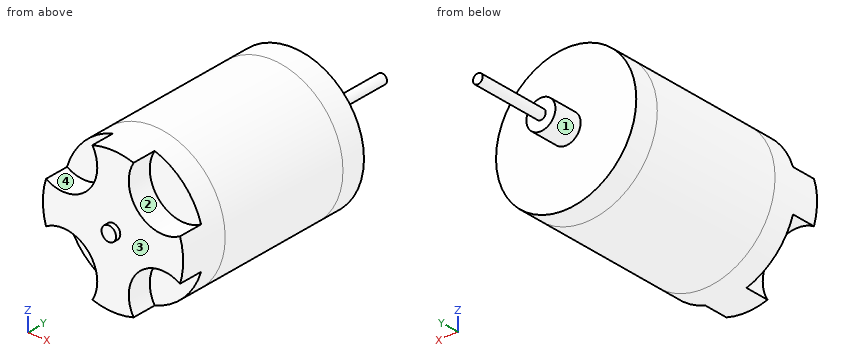
Autodesk Fusion 360 part; units mm, degrees
sketch "Sketch1" plane through (0, 0, 0) normal (0, 1, 0) x (1, 0, 0)
  circle A0 centre (0, 0) radius 14.5
  dimension "d1" = 29
extrude "Extrude1" add sketch "Sketch1" along normal blind 5
sketch "Sketch2" plane through (0, 0, 0) normal (0, -1, 0) x (1, 0, 0)
  circle A0 centre (0, 0) radius 14.5
  circle A1 centre (0, 0) radius 1.5
  circle A2 centre (0, 0) radius 14.5
  dimension "d4" = 3
extrude "Extrude2" add sketch "Sketch2" along normal blind 5 contours A0 A2 | A1
sketch "Sketch3" plane through (0, -5, 0) normal (0, -1, 0) x (1, 0, 0)
  circle A0 centre (0, 0) radius 14.5
  line L0 (0, 0) -> (10.253, 10.253)
  line L1 (0, 0) -> (14.5, 0) construction
  line L2 (0, 0) -> (10.253, -10.253)
  line L3 (0, 0) -> (-10.253, -10.253)
  line L4 (0, 0) -> (-10.253, 10.253)
  circle A1 centre (-10.253, -10.253) radius 7
  circle A2 centre (10.253, -10.253) radius 7
  circle A3 centre (10.253, 10.253) radius 7
  circle A4 centre (-10.253, 10.253) radius 7
  dimension "d7" = 45
  dimension "d8" = 14
  dimension "d9" = 14
  dimension "d10" = 14
  dimension "d11" = 14
extrude "Extrude3" cut sketch "Sketch3" against normal blind 5 contours A0 L0 A3 | A0 L2 A2 | A0 L0 A3 | A0 L2 A2 | A0 L4 A4 | A0 L3 A1 | A0 L3 A1 | A0 L4 A4
sketch "Sketch4" plane through (0, -5, 0) normal (0, -1, 0) x (1, 0, 0)
  arc A0 (-4.2549, -13.8617) -> (-13.8617, -4.2549) centre (-10.253, -10.253) ccw
  arc A1 (-4.2549, -13.8617) -> (4.2549, -13.8617) centre (0, 0) ccw
  arc A2 (13.8617, -4.2549) -> (4.2549, -13.8617) centre (10.253, -10.253) ccw
  arc A3 (13.8617, -4.2549) -> (13.8617, 4.2549) centre (0, 0) ccw
  arc A4 (4.2549, 13.8617) -> (13.8617, 4.2549) centre (10.253, 10.253) ccw
  arc A5 (4.2549, 13.8617) -> (-4.2549, 13.8617) centre (0, 0) ccw
  arc A6 (-13.8617, 4.2549) -> (-4.2549, 13.8617) centre (-10.253, 10.253) ccw
  arc A7 (-13.8617, 4.2549) -> (-13.8617, -4.2549) centre (0, 0) ccw
  circle A8 centre (0, 0) radius 1.5
  dimension "d14" = 3
extrude "Extrude4" add sketch "Sketch4" along normal blind 1 contours A8
sketch "Sketch5" plane through (0, 5, 0) normal (0, 1, 0) x (-1, 0, 0)
  circle A0 centre (0, 0) radius 14.5
  circle A1 centre (0, 0) radius 14.5
extrude "Extrude5" add sketch "Sketch5" along normal blind 28
sketch "Sketch6" plane through (0, 33, 0) normal (0, 1, 0) x (-1, 0, 0)
  circle A0 centre (0, 0) radius 14.5
  circle A1 centre (0, 0) radius 14.5
extrude "Extrude6" add sketch "Sketch6" along normal blind 5
sketch "Sketch7" plane through (0, 38, 0) normal (0, 1, 0) x (-1, 0, 0)
  circle A0 centre (0, 0) radius 14.5
  line L0 (0, 0) -> (10.253, -10.253)
  line L1 (0, 0) -> (14.5, 0) construction
  line L2 (0, 0) -> (-10.253, -10.253)
  line L3 (0, 0) -> (14.5, 0) construction
  line L4 (0, 0) -> (-10.253, 10.253)
  line L5 (-10.253, 10.253) -> (-6.7175, 6.7175)
  line L6 (-10.253, -10.253) -> (-6.7175, -6.7175)
  line L7 (10.253, -10.253) -> (6.7175, -6.7175)
  line L8 (10.253, 10.253) -> (8.8388, 8.8388)
  circle A1 centre (0, 0) radius 3.5
  circle A2 centre (0, 0) radius 12.5
  circle A3 centre (0, 0) radius 3
  dimension "d21" = 45
  dimension "d22" = 14.5
  dimension "d23" = 135
  dimension "d25" = 5
  dimension "d26" = 5
  dimension "d27" = 5
  dimension "d28" = 2
  dimension "d29" = 7
  dimension "d30" = 6
extrude "Extrude7" add sketch "Sketch7" along normal blind 6 contours L0 L2 A3 | L0 L4 A3 | L2 L4 A3
sketch "Sketch8" plane through (0, 44, 0) normal (0, 1, 0) x (-1, 0, 0)
  circle A0 centre (0, 0) radius 3
  circle A1 centre (0, 0) radius 1
  dimension "d33" = 2
extrude "Extrude8" add sketch "Sketch8" along normal blind 15 contours A1
equation "d8 = 0.7 cm * 2"
equation "d23 = 90 deg + 45 deg"
Read the model definition and answer for the solid it produces. Units are mm, in the model's axes. Face numbers are marked on the shaded views. Round coordinates to 2 decimals unless told otherwise and drop trailing zeros. Loops run counter-clockwise (first coordinate to the right, second up) from the corner with the lowest first, then second, coordinate; pieces in that order, holes last. Notation, with made-up numbers: (-5.5, 26) -> (1.5, 26) arc R20 cw to (1.5, 55) -> close; hole circle Ø10 at (24, 57). An arc over 180 degrees is marked (long way). One line per item, written item: value.
1) Flat-ended cylindrical pins translate along their axes: P1, Ø5.5, axis at x = -9, z = 9, coming from the -Y side; P2, Ø8.5, axis at x = 6.5, z = 7, coming from the -Y side; P3, Ø4, axis at x = -9, y = 8, coming from the -Z side. Find the tip coordinate at first contact, or state that the pin passes through.
Answer list:
P1: stops at y = 0
P2: stops at y = -5
P3: stops at z = -12.7
2) The mould has two halves that part along X. Classify the marked faces 1, 2, 3 and 4: pulls with the +X half, pulls with the -X half, needs draft (parallel to the pull), parting line crosses it, or undercut.
Answer list:
face 1: parting line crosses it
face 2: undercut
face 3: needs draft
face 4: undercut
3) A cutting plane is placed at C-C (y = 37). Determine the outline of the cut face in (x, z).
Answer list:
outline: circle Ø29 at (0, 0)
4) A cutting plane is placed at A-A (x = 0). Determine the outline of the cut face in (y, z).
Answer list:
outline: (-6, -1.5) -> (-5, -1.5) -> (-5, -14.5) -> (38, -14.5) -> (38, -3) -> (44, -3) -> (44, -1) -> (59, -1) -> (59, 1) -> (44, 1) -> (44, 3) -> (38, 3) -> (38, 14.5) -> (-5, 14.5) -> (-5, 1.5) -> (-6, 1.5) -> close
5) A cutting plane is placed at B-B (z = 8). Determine the outline of the cut face in (x, y), and give its area (3 significant figures).
Answer list:
outline: (-12.09, 0) -> (-3.63, 0) -> (-3.63, -5) -> (3.63, -5) -> (3.63, 0) -> (12.09, 0) -> (12.09, 38) -> (-12.09, 38) -> close
area: 955 mm²
6) A cutting plane is placed at D-D (x = -7.25). Determine the outline of the cut face in (y, z), and give its area (3 significant figures).
Answer list:
outline: (-5, -3.93) -> (0, -3.93) -> (0, -12.56) -> (38, -12.56) -> (38, 12.56) -> (0, 12.56) -> (0, 3.93) -> (-5, 3.93) -> close
area: 994 mm²
7) Consider L1, parallel to Y at x = 4.75, z = 7; L2, parallel to Y at x = 9.5, z = 1.5; L3, parallel to X at y = 12.5, z = -1. Determine where each line is inside the solid, lowest interval first. Write a range as [from, to].
Answer list:
L1: y = [0, 38]
L2: y = [-5, 38]
L3: x = [-14.47, 14.47]
